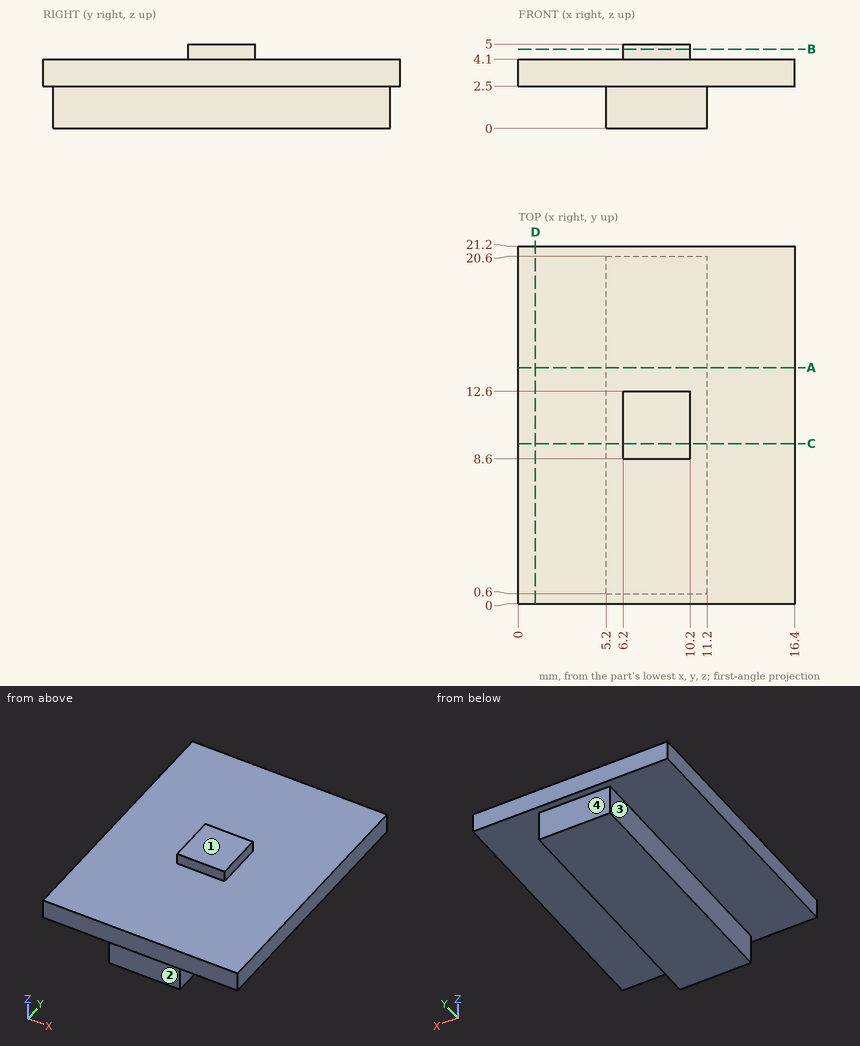
Geometry: see drawing. Coordinates: mm, zero at the bounding-box minimum. A direction names the side the tool comes from. Give positions to 0.01 mm unless a question says otherwise; leave off trailing zeros. Loops run counter-clockwise (first coordinate to the right, second up) from the corner with the lowest first, then second, coordinate; pieces in that order, holes last. Notation, with made-up numbers: (68, 1) -> (124, 1) arc R24 ccw to (124, 17) -> close; hole circle Ø11 at (63, 24.25). An arc over 180 degrees is marked (long way). Answer as a JSON object with one key per item and string values. Group by question number.
Item 1: Cut plane C-C, the plane y = 9.5. Return the cut outline in (x, z).
Item 2: Pin query (flat end, axial travel): P1, Ø1.5, axis at x = 6, y = 13.5, coming from the +Z side; P2, Ø0.8, axis at y = 7, z = 2, coming from the +X side; P3, Ø0.5, axis at x = 7, z = 4.5, coming from the +Y side; P4, Ø1, axis at x = 13.5, z = 0.5, coming from the +Y side. Return the tip coordinate at first contact, or that it passes through.
Item 3: Reachability of the marked faces 1, 2, 3 and 4 from +Z, -Z, +X, -X, +Y, -Y: full face, straight path, thin tool, end or side. Return the list, or none.
Item 4: Line query: probe 1 along Z at (x, y) = (8, 14.5); probe 2 along Z at (x, y) = (2, 9.75); probe 3 along X at (y, z) = (6.75, 2). Output: solid intervals per line, ascending.
Item 5: Cut plane D-D, the plane x = 1. Return the cut outline in (y, z).
Item 6: Cut plane B-B, the plane z = 4.7. Return the cut outline in (x, y), and give its area (3 significant figures).
Item 7: Cut plane A-A, the plane y = 14. Return the cut outline in (x, z).
Checks:
{
 "1": {"outline": "(0, 2.5) -> (5.2, 2.5) -> (5.2, 0) -> (11.2, 0) -> (11.2, 2.5) -> (16.4, 2.5) -> (16.4, 4.1) -> (10.2, 4.1) -> (10.2, 5) -> (6.2, 5) -> (6.2, 4.1) -> (0, 4.1) -> close"},
 "2": {"P1": "stops at z = 4.1", "P2": "stops at x = 11.2", "P3": "stops at y = 12.6", "P4": "passes through"},
 "3": {"face 1": "+Z, +X, -X, +Y, -Y", "face 2": "-Z, +X, -X, -Y", "face 3": "-Z, -X, +Y, -Y", "face 4": "-Z, +X, -X, +Y"},
 "4": {"probe 1": "z = 0 to 4.1", "probe 2": "z = 2.5 to 4.1", "probe 3": "x = 5.2 to 11.2"},
 "5": {"outline": "(0, 2.5) -> (21.2, 2.5) -> (21.2, 4.1) -> (0, 4.1) -> close"},
 "6": {"outline": "(6.2, 8.6) -> (10.2, 8.6) -> (10.2, 12.6) -> (6.2, 12.6) -> close", "area": "16.0 mm²"},
 "7": {"outline": "(0, 2.5) -> (5.2, 2.5) -> (5.2, 0) -> (11.2, 0) -> (11.2, 2.5) -> (16.4, 2.5) -> (16.4, 4.1) -> (0, 4.1) -> close"}
}
